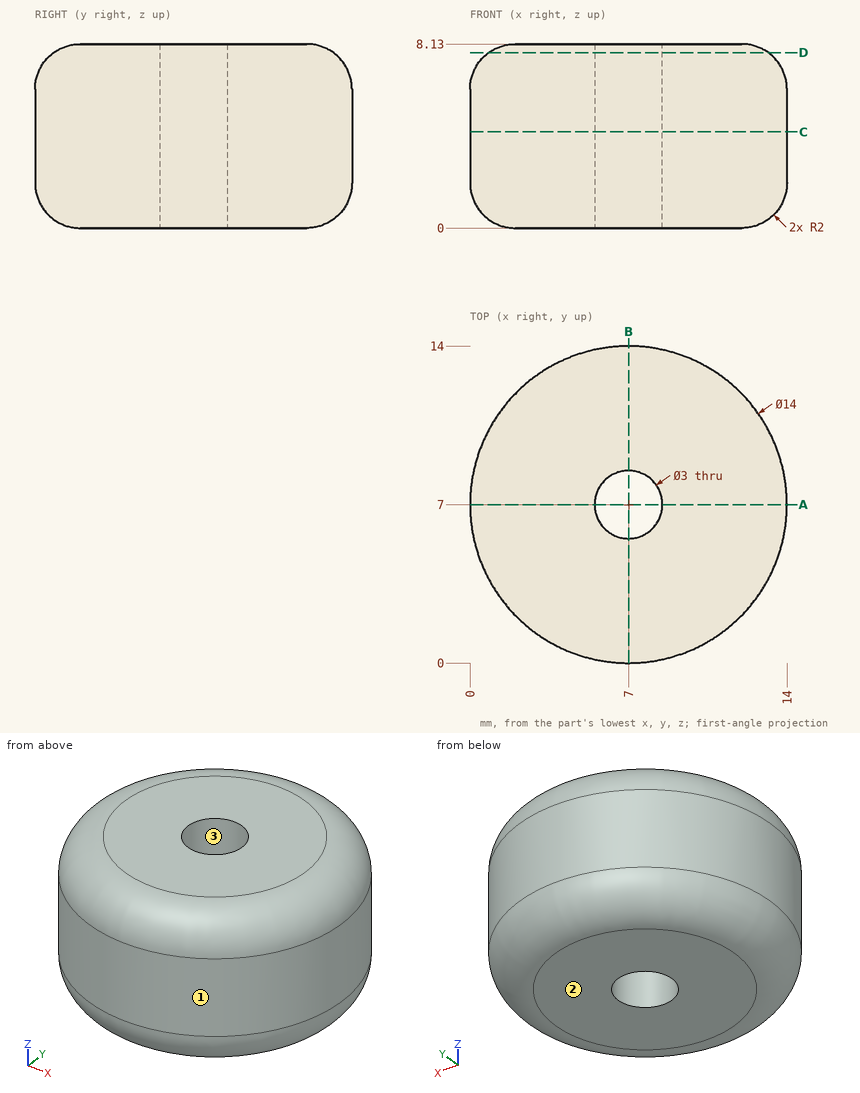
Verification items for this drawing (mm, ordinates from the low corner). Give positions to 0.01 mm unless a question says otherwise; leave off trailing zeros. Loops run counter-clockwise (first coordinate to the right, second up) from the corner with the lowest first, then second, coordinate; pieces in that order, holes last.
(1) Section check D-D on z = 7.75. Record the cut outline in (x, y).
From the geometry:
outline: circle Ø12.35 at (7, 7); hole circle Ø3 at (7, 7)
(2) Depth check by flat-ended pin: pin 1 Ø1.5 at (y, z) = (10, 6.5) entering from +X; pin 2 Ø2 at (x, z) = (11, 4.5) entering from -Y. Enter the tip coordinate at first touch or a pass-through.
From the geometry:
pin 1: stops at x = 13.61
pin 2: stops at y = 0.68
(3) Thickness scan on L1, parallel to Y at x = 7, z = 3; L2, parallel to X at y = 6.75, z = 0.75; L3, parallel to Y at x = 6, z = 4.5. Record the ranges inside material, lowest first.
From the geometry:
L1: y = 0 to 5.5, 8.5 to 14
L2: x = 0.44 to 5.52, 8.48 to 13.56
L3: y = 0.07 to 5.88, 8.12 to 13.93
(4) Section check A-A on y = 7. Record the cut outline in (x, z).
From the geometry:
outline: (0, 2) arc R2 ccw to (2, 0) - (5.5, 0) - (5.5, 8.13) - (2, 8.13) arc R2 ccw to (0, 6.13) - close; (8.5, 0) - (12, 0) arc R2 ccw to (14, 2) - (14, 6.13) arc R2 ccw to (12, 8.13) - (8.5, 8.13) - close
(5) Release check for a two-part mould opening along Y. For the marked faces 1, 2 and 3 record: released by +Y, released by -Y, zero draft, split by the parting line, or undercut.
From the geometry:
face 1: split by the parting line
face 2: zero draft
face 3: undercut
(6) Section check C-C on z = 4.25. Record the cut outline in (x, y).
From the geometry:
outline: circle Ø14 at (7, 7); hole circle Ø3 at (7, 7)
